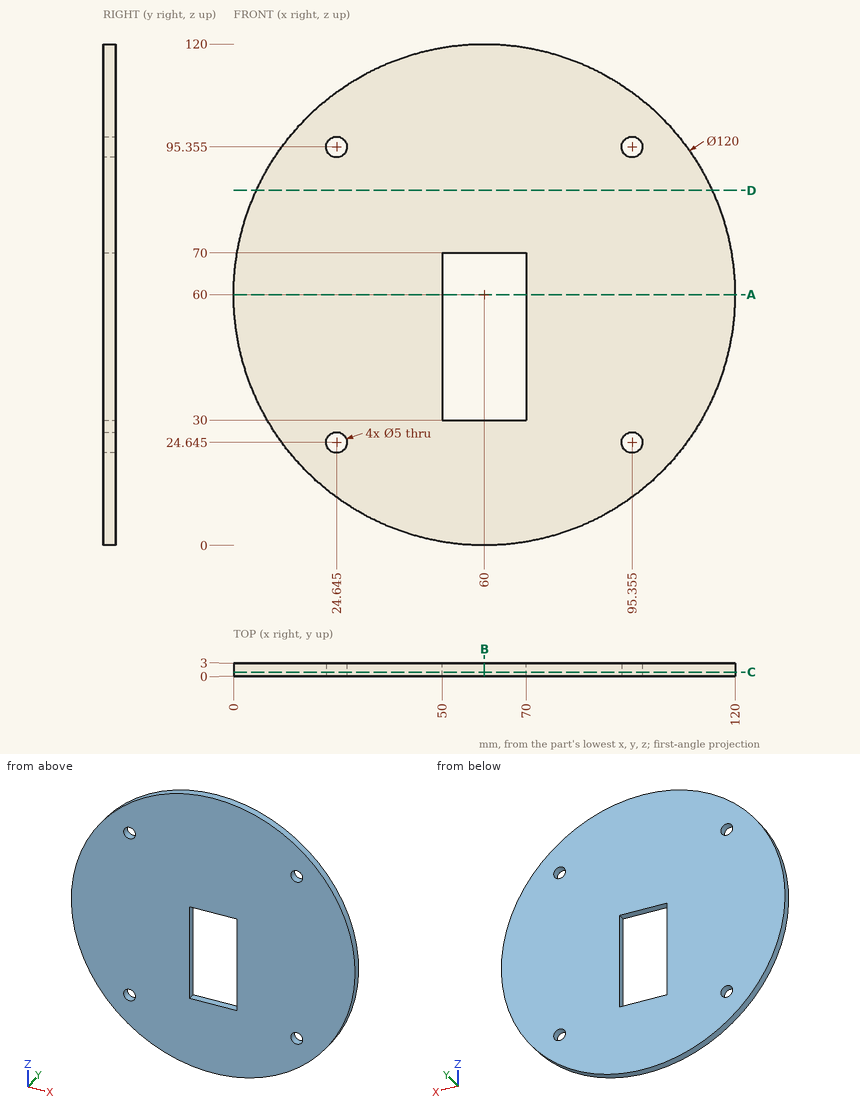
Geometry: see drawing. Coordinates: mm, zero at the bounding-box minimum. Give positions to 0.01 mm unless a question says otherwise; leave off trailing zeros. Write each loop counter-clockwise with the first axis right and the second up, starting at its lowest first coordinate (ties: lowest second). Pieces come first, ordered by that corner, then holes. Notation, with made-up numbers: M -10,-5 L 9,-5 A7 ccw 9,3 Z; hole C 47,89 d1. An arc over 180 degrees is marked long. Return JSON: item names as keys, results as strings. Group by question number.
1) Cut plane B-B, the plane x = 60. Output: boundary loops of the cut face in (y, z), then the cut area to 3 significant figures.
2) Cut plane C-C, the plane y = 0.9. Output: boundary loops of the cut face in (x, z) (1 decimal), then the cut area to 3 significant figures.
3) Ray query, L1, parallel to Z at x = 59, y = 1.2; L2, parallel to X at y = 1.95, z = 94.5 (1 decimal); L3, parallel to X at y = 2.2, z = 60. Return the intervals inside material, ascending.
4) Cut plane A-A, the plane z = 60. Output: boundary loops of the cut face in (x, y).
5) First-contact query: pin 1 Ø4 at (x, z) = (95.36, 24.64) entering from -Y; pin 2 Ø1.5 at (y, z) = (1.5, 97.5) entering from +X; pin 3 Ø1.5 at (y, z) = (0.5, 38.5) entering from +X; pin 4 Ø0.9 at (x, y) = (58.5, 1) entering from +Z. Flat tips, straight axial feed; report the tip coordinate or a pass-through.
6) Cut plane D-D, the plane z = 85. Output: boundary loops of the cut face in (x, y).
Data:
{
 "1": {"outline": "M 0,0 L 3,0 L 3,30 L 0,30 Z; M 0,70 L 3,70 L 3,120 L 0,120 Z", "area": "240 mm²"},
 "2": {"outline": "C 60,60 d120; hole C 24.6,24.6 d5; hole C 24.6,95.4 d5; hole M 50,30 L 70,30 L 70,70 L 50,70 Z; hole C 95.4,24.6 d5; hole C 95.4,95.4 d5", "area": "10,400 mm²"},
 "3": {"L1": "z = 0.01 to 30, 70 to 119.99", "L2": "x = 10.9 to 22.3, 27 to 93, 97.7 to 109.1", "L3": "x = 0 to 50, 70 to 120"},
 "4": {"outline": "M 0,0 L 50,0 L 50,3 L 0,3 Z; M 70,0 L 120,0 L 120,3 L 70,3 Z"},
 "5": {"pin 1": "passes through", "pin 2": "stops at x = 107.43", "pin 3": "stops at x = 116.3", "pin 4": "stops at z = 119.99"},
 "6": {"outline": "M 5.46,0 L 114.54,0 L 114.54,3 L 5.46,3 Z"}
}
